```python
from build123d import *

# Parameters (mm, degrees)
SKETCH1_R           = 34.25
SKETCH1_R_2         = 29.25
BOSS_EXTRUDE1_DEPTH = 20
SKETCH2_R           = 1.5
CUT_EXTRUDE1_DEPTH  = 20
CIRPATTERN1_COUNT   = 4
FILLET1_R           = 1


with BuildPart() as part:
    # Sketch1 → Boss-Extrude1 (new body)
    with BuildSketch(Plane(origin=(0, 0, 0), x_dir=(1, 0, 0), z_dir=(0, 1, 0))):
        with Locations(Location((0, 0, 0), (0, 0, 270))):
            Circle(SKETCH1_R)
        with Locations(Location((0, 0, 0), (0, 0, 270))):
            Circle(SKETCH1_R_2, mode=Mode.SUBTRACT)
    extrude(amount=BOSS_EXTRUDE1_DEPTH)

    # Sketch2 → Cut-Extrude1 (cut)
    with BuildSketch(Plane.ZY.offset(34.25)):
        with Locations((0, 10)):
            Circle(SKETCH2_R)
    cut_extrude1 = extrude(amount=-CUT_EXTRUDE1_DEPTH, mode=Mode.SUBTRACT)

    # CirPattern1: Cut-Extrude1 ×4 about axis
    cirpattern1_axis = Axis((0, 20, 0), (0, -1, 0))
    for i in range(1, CIRPATTERN1_COUNT):
        add(cut_extrude1.rotate(cirpattern1_axis, i * 360 / CIRPATTERN1_COUNT), mode=Mode.SUBTRACT)

    # Fillet1
    fillet1_edges = [part.edges().sort_by_distance(p)[0] for p in [
        (0, 20, -29.25),
    ]]
    fillet(fillet1_edges, radius=FILLET1_R)


solid = part.part
```
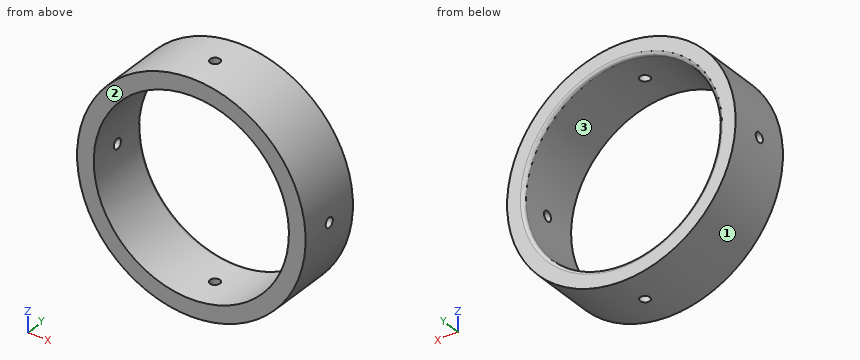
Design review of the part built by this model. Coordinates are the model's own, in mm. Face numbers are marked on the shaded views. Round coordinates to 2 decimals unless told otherwise and drop trailing zeros. Write each loop counter-clockwise with the first axis right and the second up, starting at its lowest first coordinate (ties: lowest second). Pieces come first, ordered by that corner, then holes.
Item 1: For probe 1 along Z at (x, y) = (0, 5.5); probe 2 along Y at (x, z) = (0, 31), list the stretches that pass through material, from the lowest coordinate up.
Item 2: We need section C-C on y = 10. Write out the cut boundary in (x, z), and give its area (3 significant figures).
Item 3: Clearance check with flat-ended pins moving along their axes: pin 1 Ø3 at (x, y) = (-6, 14.5) entering from -Z; pin 2 Ø5 at (x, y) = (0, 10) entering from -Z; pin 3 Ø3 at (y, z) = (16, -8) entering from -X; pin 4 Ø4 at (y, z) = (3.5, 4.5) entering from +X. State where each tip first meets the part, or that it passes through.
Item 4: We need section B-B on z = 0. Write out the cut boundary in (x, y).
Item 5: We need section D-D on y = 3.75. Write out the cut boundary in (x, z).
Item 6: The part is to be moulded in two halves that separate along X. For the marked faces 1, 2 and 3, say which applies: +X half, -X half, draft (parallel to the pull), parting line (faces both ways), or undercut.
Item 7: We need section A-A on x = 0. Write out the cut boundary in (y, z).
Returned:
1. probe 1: z = -34.25 to -29.25, 29.25 to 34.25
1. probe 2: y = 0 to 8.5, 11.5 to 20
2. outline: (-34.22, -1.5) arc R34.25 ccw to (-1.5, -34.22) - (-1.5, -29.21) arc R29.25 cw to (-29.21, -1.5) - close; (-34.22, 1.5) - (-29.21, 1.5) arc R29.25 cw to (-1.5, 29.21) - (-1.5, 34.22) arc R34.25 ccw to start; (1.5, -34.22) arc R34.25 ccw to (34.22, -1.5) - (29.21, -1.5) arc R29.25 cw to (1.5, -29.21) - close; (1.5, 29.21) arc R29.25 cw to (29.21, 1.5) - (34.22, 1.5) arc R34.25 ccw to (1.5, 34.22) - close
2. area: 937 mm2
3. pin 1: stops at z = -33.95
3. pin 2: stops at z = -34.25
3. pin 3: stops at x = -33.63
3. pin 4: stops at x = 34.16
4. outline: (-34.25, 0) - (-29.25, 0) - (-29.25, 8.5) - (-34.25, 8.5) - close; (-34.25, 11.5) - (-29.25, 11.5) - (-29.25, 19) arc R1 ccw to (-30.25, 20) - (-34.25, 20) - close; (29.25, 0) - (34.25, 0) - (34.25, 8.5) - (29.25, 8.5) - close; (29.25, 11.5) - (34.25, 11.5) - (34.25, 20) - (30.25, 20) arc R1 ccw to (29.25, 19) - close
5. outline: circle Ø68.5 at (0, 0); hole circle Ø58.5 at (0, 0)
6. face 1: parting line
6. face 2: draft
6. face 3: undercut
7. outline: (0, -34.25) - (8.5, -34.25) - (8.5, -29.25) - (0, -29.25) - close; (0, 29.25) - (8.5, 29.25) - (8.5, 34.25) - (0, 34.25) - close; (11.5, -34.25) - (20, -34.25) - (20, -30.25) arc R1 ccw to (19, -29.25) - (11.5, -29.25) - close; (11.5, 29.25) - (19, 29.25) arc R1 ccw to (20, 30.25) - (20, 34.25) - (11.5, 34.25) - close
